```python
from build123d import *

# Parameters (mm, degrees)
PAD_DEPTH       = 1.65
SKETCH001_R     = 3.675
PAD001_DEPTH    = 2.2
SKETCH002_R     = 1.65
POCKET_DEPTH    = 2.6
SKETCH003_R     = 2.4
POCKET001_DEPTH = 0.8
SKETCH004_R     = 1.2
POCKET002_DEPTH = 3.051


with BuildPart() as part:
    # Sketch → Pad (new body)
    with BuildSketch(Plane.XY):
        with BuildLine():
            Line((-1.795904, 17.921356), (-2.85, 2.320156))
            ThreePointArc((-2.85, 2.320156), (0, -3.675), (2.85, 2.320156))
            Line((1.795904, 17.921356), (2.85, 2.320156))
            ThreePointArc((1.795904, 17.921356), (0, 19.6), (-1.795904, 17.921356))
        make_face()
    extrude(amount=-PAD_DEPTH)

    # Sketch001 → Pad001 (new body)
    with BuildSketch(Plane(origin=(0, 0, -1.65), x_dir=(1, 0, 0), z_dir=(0, 0, -1))):
        Circle(SKETCH001_R)
    extrude(amount=PAD001_DEPTH)

    # Sketch002 → Pocket (cut)
    with BuildSketch(Plane(origin=(0, 0, -3.85), x_dir=(1, 0, 0), z_dir=(0, 0, -1))):
        Circle(SKETCH002_R)
    extrude(amount=-POCKET_DEPTH, mode=Mode.SUBTRACT)

    # Sketch003 → Pocket001 (cut)
    with BuildSketch(Plane.XY):
        Circle(SKETCH003_R)
    extrude(amount=-POCKET001_DEPTH, mode=Mode.SUBTRACT)

    # Sketch004 → Pocket002 (cut, through all)
    with BuildSketch(Plane.XY.offset(-0.8)):
        Circle(SKETCH004_R)
    extrude(amount=-POCKET002_DEPTH, mode=Mode.SUBTRACT)


solid = part.part
```
Design review of the part built by this model. Coordinates are the model's own, in mm. A direction names the side the tool comes from. Round coordinates to 2 decimals unless told otherwise and drop trailing zeros. Order: outer loops, then holes, each group sorted by start corner. A loop starts at its lowest first (then second) coordinate and runs counter-clockwise, first axis right, second up. Notation, with made-up numbers: (-26, 10) - (-3, 10) arc R7 cw to (-3, 21) - close; hole circle Ø3 at (58.5, -16.75). An arc over 180 degrees is marked (long way). One line per question, with ' | ' between items.
Item 1: Take a section at D-D, the plane x = 2. Write out the cut boundary in (y, z), then the cut area to 3 significant figures.
Checks:
outline: (-3.08, -3.85) - (3.08, -3.85) - (3.08, -1.65) - (14.9, -1.65) - (14.9, 0) - (1.33, 0) - (1.33, -0.8) - (-1.33, -0.8) - (-1.33, 0) - (-3.08, 0) - close | area: 41.1 mm²
Item 2: Take a section at C-C, the plane x = 0. Write out the cut boundary in (y, z) (3 decimals), then the cut area to 3 significant figures.
Checks:
outline: (-3.675, -3.85) - (-1.65, -3.85) - (-1.65, -1.25) - (-1.2, -1.25) - (-1.2, -0.8) - (-2.4, -0.8) - (-2.4, 0) - (-3.675, 0) - close; (1.2, -1.25) - (1.65, -1.25) - (1.65, -3.85) - (3.675, -3.85) - (3.675, -1.65) - (19.6, -1.65) - (19.6, 0) - (2.4, 0) - (2.4, -0.8) - (1.2, -0.8) - close | area: 41.1 mm²
Item 3: Wall thickness on line 1 (Y direction, x = 0, z = -2.15) (3 decimals); line 2 (Y direction, x = 0, z = -1.1) (3 decimals): over which ranges is each line inside the solid? List them lowest first. Write a range as [from, to].
Checks:
line 1: [-3.675, -1.65], [1.65, 3.675] | line 2: [-3.675, -1.2], [1.2, 19.6]
Item 4: Take a section at B-B, the plane z = -0.6. Write out the cut boundary in (x, y) (3 decimals).
Checks:
outline: (-2.85, 2.32) arc R3.675 ccw (long way) to (2.85, 2.32) - (1.796, 17.921) arc R1.8 ccw to (-1.796, 17.921) - close; hole circle Ø4.8 at (0, 0)
Item 5: Take a section at A-A, the plane y = 0. Write out the cut boundary in (x, z) (3 decimals).
Checks:
outline: (-3.675, -3.85) - (-1.65, -3.85) - (-1.65, -1.25) - (-1.2, -1.25) - (-1.2, -0.8) - (-2.4, -0.8) - (-2.4, 0) - (-3.675, 0) - close; (1.2, -1.25) - (1.65, -1.25) - (1.65, -3.85) - (3.675, -3.85) - (3.675, 0) - (2.4, 0) - (2.4, -0.8) - (1.2, -0.8) - close
Item 6: Draft analysis for pull direction X (two halves, no side actions). For faces 1 (the face through (-2.316, 10.23, -0.813)), 2 (the face through (0, 11, -1.65)), 3 (the face through (-1.216, -1.115, -2.568)), 4 (the face through (-1, 1, -0.8)), state which applies: +X half, -X half, draft (parallel to the pull), parting line (faces both ways), or undercut.
Checks:
face 1: -X half | face 2: draft | face 3: undercut | face 4: undercut
Item 7: For P1, Ø1, axis at x = 1.5, z = -2.5, coming from the -Y side; P2, Ø2, axis at y = 7, z = -1, coming from the +X side; P3, Ø4, axis at x = -2.5, y = 14, coming from the -Z side, all flat-tipped, find the tip position at first contact; note any pin that passes through.
Checks:
P1: y = -3.54 | P2: x = 2.6 | P3: z = -1.65
Item 8: Machinability: for faces 5 (the face through (0.65, 1.01, -1.02)), 6 (the face through (1, 1, -1.25)), 7 (the face through (1.29, 2.024, -0.394)), which of the approach directions +Z, -Z, +X, -X, +Y, -Y give a long, thin tool a straight path to every point of the face, cutting with its end or side? Answer none if there is none.
Checks:
face 5: +Z, -Z | face 6: -Z | face 7: +Z
